```python
from build123d import *

# Parameters (mm, degrees)
SKETCH3_R           = 19.05
SKETCH3_R_2         = 12.7
SKETCH4_R           = 44.45
SKETCH4_R_2         = 3.175
BOSS_EXTRUDE1_DEPTH = 6.35


with BuildPart() as part:
    # Sweep1: sweep along a path in Sketch1
    with BuildLine(Plane.XY) as sweep1_path:
        ThreePointArc((76.2, 0), (52.411249779, 55.31275528), (-4.101860805, 76.089517924))
    # Sketch3 → Sweep1 (sweep)
    with BuildSketch(Plane(origin=(0, 0, 0), x_dir=(1, 0, 0), z_dir=(0, 1, 0))):
        with Locations((76.2, 0)):
            Circle(SKETCH3_R)
        with Locations((76.2, 0)):
            Circle(SKETCH3_R_2, mode=Mode.SUBTRACT)
    sweep(path=sweep1_path.line)

    # Sketch4 → Boss-Extrude1 (add)
    with BuildSketch(Plane.XZ):
        with Locations((76.2, 0)):
            Circle(SKETCH4_R)
        with Locations((76.2, 31.75)):
            Circle(SKETCH4_R_2, mode=Mode.SUBTRACT)
        with Locations((107.95, 0)):
            Circle(SKETCH4_R_2, mode=Mode.SUBTRACT)
        with Locations((76.2, -31.75)):
            Circle(SKETCH4_R_2, mode=Mode.SUBTRACT)
        with Locations((44.45, 0)):
            Circle(SKETCH4_R_2, mode=Mode.SUBTRACT)
    boss_extrude1 = extrude(amount=BOSS_EXTRUDE1_DEPTH)

    # Mirror1: Boss-Extrude1 across plane
    add(boss_extrude1.mirror(Plane(origin=(0, 0, 0), x_dir=(0, 0, 1), z_dir=(-0.707106781, 0.707106781, 0))))


solid = part.part
```
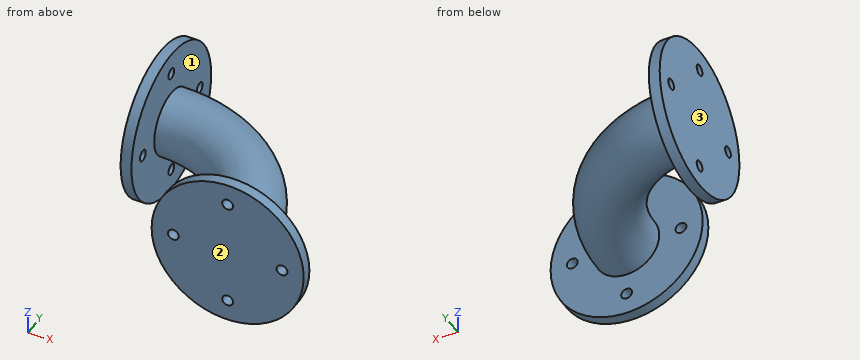
Can you work these out from the model? Positions are in its coordinate system, mm. Face numbers are marked on the shaded views. Give positions to 0.01 mm unless a question says otherwise; leave off trailing zeros. Loops run counter-clockwise (first coordinate to the right, second up) from the corner with the lowest first, then second, coordinate; pieces in that order, holes last. Notation, with made-up numbers: M 11.25,-30.5 L 58.25,-30.5 A8 cw 58.25,-21.5 Z; hole C -29,58 d10. An arc over 180 degrees is marked long. Use one line per item in the form item = value. Start each with the question number.
(1) Please list where these lines run through material, in increasing order: line 1 (Z direction, x = 76.2, y = -1.75) (3 decimals); line 2 (X direction, y = 46, z = 3); line 3 (X direction, y = 99.5, z = 19.5).
(2) I want a section at B-B, the plane z = 31.75. Write out the boundary of the cut face in (x, y) (3 decimals).
(3) Thinking about a two-plate mould opening in X: for the marked faces 1, 2 and 3, which applies, released by +X, released by -X, zero draft, split by the parting line, or undercut?
(4) I want a section at C-C, the plane y = 109. Write out the boundary of the cut face in (x, z), and give its area (3 significant figures).
(5) I'm going to push flat-ended pins straight in: P1, Ø5, axis at y = 44.45, z = 0, coming from the -X side; P2, Ø4, axis at x = 74, y = 10, coming from the +Z side; P3, Ø5, axis at x = 37.5, y = 82, coming from the +Z side. Where does each tip first touch, or does it pass through?
(6) I want a section at A-A, the plane y = 76.2. State how many separate pieces and enclosed holes the cut face has, and give its area (3 significant figures).
Worked out:
q1.line_1 = -44.45 to -34.925, -28.575 to 28.575, 34.925 to 44.45
q1.line_2 = -6.35 to 0, 34.31 to 44.29, 75.65 to 83.13
q1.line_3 = -6.35 to 0
q2.outline = M -6.35,45.091 L 0,45.091 L 0,73.025 L -6.35,73.025 Z; M -6.35,79.375 L 0,79.375 L 0,107.309 L -6.35,107.309 Z; M 45.091,-6.35 L 73.025,-6.35 L 73.025,0 L 45.091,0 Z; M 79.375,-6.35 L 107.309,-6.35 L 107.309,0 L 79.375,0 Z
q3.face_1 = undercut
q3.face_2 = zero draft
q3.face_3 = released by -X
q4.outline = M -6.35,-30 L 0,-30 L 0,-3 L -6.35,-3 Z; M -6.35,3 L 0,3 L 0,30 L -6.35,30 Z
q4.area = 343 mm²
q5.P1 = 32.59
q5.P2 = 19.05
q5.P3 = 15.21
q6.separate_pieces = 3
q6.enclosed_holes = 1
q6.area = 1,360 mm²
